```python
from build123d import *

# Parameters (mm, degrees)
BOSS_EXTRUDE1_DEPTH = 24
SKETCH2_R           = 10.5
CUT_EXTRUDE1_DEPTH  = 2.5
SKETCH4_R           = 2.25
SKETCH4_R_2         = 1.25
CUT_EXTRUDE2_DEPTH  = 10
SKETCH11_R          = 3
BOSS_EXTRUDE2_DEPTH = 4
CUT_EXTRUDE5_DEPTH  = 65
SKETCH13_W          = 24
SKETCH13_H          = 8.6
SKETCH13_R          = 2.2
BOSS_EXTRUDE3_DEPTH = 5
SKETCH14_W          = 5
SKETCH14_H          = 15
BOSS_EXTRUDE4_DEPTH = 7.5
SKETCH15_W          = 3
SKETCH15_H          = 15
BOSS_EXTRUDE5_DEPTH = 20
SKETCH16_R          = 5.05
CUT_EXTRUDE6_DEPTH  = 79.900823823
CHAMFER1_SIZE       = 3
CHAMFER2_SIZE       = 1
FILLET2_R           = 6
FILLET7_R           = 3
FILLET8_R           = 0.5


with BuildPart() as part:
    # Sketch1 → Boss-Extrude1 (new body)
    with BuildSketch(Plane(origin=(0, 0, 0), x_dir=(0, 0, -1), z_dir=(1, 0, 0))):
        Polygon((0, 59.7), (0, 0), (-43, 0), (-43, 5), (-8.535533906, 5), (-5, 8.535533906), (-5, 51.164466094), (-8.535533906, 54.7), (-43, 54.7), (-43, 59.7), align=None)
    extrude(amount=BOSS_EXTRUDE1_DEPTH)

    # Sketch2 → Cut-Extrude1 (cut)
    with BuildSketch(Plane.XZ.offset(-54.7)):
        with Locations(Location((12, 31, 0), (0, 0, 270))):
            Circle(SKETCH2_R)
    extrude(amount=-CUT_EXTRUDE1_DEPTH, mode=Mode.SUBTRACT)

    # Sketch4 → Cut-Extrude2 (cut)
    with BuildSketch(Plane.XZ.offset(-57.2)):
        with Locations(Location((12, 31, 0), (0, 0, 270))):
            Circle(SKETCH4_R)
        with Locations(Location((12, 38.25, 0), (0, 0, 270))):
            Circle(SKETCH4_R_2)
        with Locations(Location((8.5, 38.25, 0), (0, 0, 270))):
            Circle(SKETCH4_R_2)
        with Locations(Location((15.5, 38.25, 0), (0, 0, 270))):
            Circle(SKETCH4_R_2)
        with Locations(Location((19.25, 34.5, 0), (0, 0, 270))):
            Circle(SKETCH4_R_2)
        with Locations(Location((19.25, 31, 0), (0, 0, 270))):
            Circle(SKETCH4_R_2)
        with Locations(Location((19.25, 27.5, 0), (0, 0, 270))):
            Circle(SKETCH4_R_2)
        with Locations(Location((15.5, 23.75, 0), (0, 0, 270))):
            Circle(SKETCH4_R_2)
        with Locations(Location((12, 23.75, 0), (0, 0, 270))):
            Circle(SKETCH4_R_2)
        with Locations(Location((8.5, 23.75, 0), (0, 0, 270))):
            Circle(SKETCH4_R_2)
        with Locations(Location((4.75, 27.5, 0), (0, 0, 270))):
            Circle(SKETCH4_R_2)
        with Locations(Location((4.75, 31, 0), (0, 0, 270))):
            Circle(SKETCH4_R_2)
        with Locations(Location((4.75, 34.5, 0), (0, 0, 270))):
            Circle(SKETCH4_R_2)
    extrude(amount=-CUT_EXTRUDE2_DEPTH, mode=Mode.SUBTRACT)

    # Sketch11 → Boss-Extrude2 (add)
    with BuildSketch(Plane(origin=(0, 5, 0), x_dir=(1, 0, 0), z_dir=(0, 1, 0))):
        with Locations(Location((12, -31, 0), (0, 0, 90))):
            Circle(SKETCH11_R)
    extrude(amount=BOSS_EXTRUDE2_DEPTH)

    # Sketch12 → Cut-Extrude5 (cut, symmetric)
    with BuildSketch(Plane.XZ.offset(-54.7)):
        with BuildLine():
            Line((6, 12.017766953), (18, 12.017766953))
            ThreePointArc((18, 12.017766953), (20.5, 14.517766953), (18, 17.017766953))
            Line((18, 17.017766953), (6, 17.017766953))
            ThreePointArc((6, 17.017766953), (3.5, 14.517766953), (6, 12.017766953))
        make_face()
    extrude(amount=CUT_EXTRUDE5_DEPTH, both=True, mode=Mode.SUBTRACT)

    # Sketch13 → Boss-Extrude3 (add)
    # profile 1 of 2: a face of its own
    with BuildSketch(Plane.ZY):
        with Locations((-12, 4.3)):
            Rectangle(SKETCH13_W, SKETCH13_H)
        with Locations((-16.95, 4.3)):
            Circle(SKETCH13_R, mode=Mode.SUBTRACT)
        with Locations((-7.05, 4.3)):
            Circle(SKETCH13_R, mode=Mode.SUBTRACT)
    # profile 2 of 2: a face of its own
    with BuildSketch(Plane.ZY):
        with Locations((-12, 53.4)):
            Rectangle(SKETCH13_W, SKETCH13_H)
        with Locations(Location((-16.95, 53.4, 0), (0, 0, 180))):
            Circle(SKETCH13_R, mode=Mode.SUBTRACT)
        with Locations(Location((-7.05, 53.4, 0), (0, 0, 180))):
            Circle(SKETCH13_R, mode=Mode.SUBTRACT)
    extrude(amount=-BOSS_EXTRUDE3_DEPTH)

    # Sketch14 → Boss-Extrude4 (add)
    with BuildSketch(Plane(origin=(24, 0, 0), x_dir=(0, 0, -1), z_dir=(1, 0, 0))):
        with Locations((-2.5, 17.6)):
            Rectangle(SKETCH14_W, SKETCH14_H)
    extrude(amount=BOSS_EXTRUDE4_DEPTH)

    # Sketch15 → Boss-Extrude5 (add)
    with BuildSketch(Plane(origin=(0, 0, 0), x_dir=(-1, 0, 0), z_dir=(0, 0, -1))):
        with Locations((-30, 17.6)):
            Rectangle(SKETCH15_W, SKETCH15_H)
    extrude(amount=BOSS_EXTRUDE5_DEPTH)

    # Sketch16 → Cut-Extrude6 (cut, through all)
    with BuildSketch(Plane.ZY.offset(-28.5)):
        with Locations((-12, 17.6)):
            Circle(SKETCH16_R)
    extrude(amount=-CUT_EXTRUDE6_DEPTH, mode=Mode.SUBTRACT)

    # Chamfer1
    chamfer1_edges = [part.edges().sort_by_distance(p)[0] for p in [
        (24, 25.1, 2.5),
    ]]
    chamfer(chamfer1_edges, length=CHAMFER1_SIZE)

    # Chamfer2
    chamfer2_edges = [part.edges().sort_by_distance(p)[0] for p in [
        (24, 10.1, 2.5),
    ]]
    chamfer(chamfer2_edges, length=CHAMFER2_SIZE)

    # Fillet2
    fillet2_edges = [part.edges().sort_by_distance(p)[0] for p in [
        (0, 2.5, 43),
        (0, 57.2, 43),
        (24, 2.5, 43),
        (24, 57.2, 43),
    ]]
    fillet(fillet2_edges, radius=FILLET2_R)

    # Fillet7
    # the kernel refuses this fillet: 3 mm, written as the material it takes off along each edge
    with BuildSketch(Plane(origin=(-7.5, 59.7, 0), x_dir=(0, -1, 0), z_dir=(1, 0, 0))) as fillet7_piece_1_section:
        with BuildLine():
            CenterArc((FILLET7_R, -FILLET7_R), FILLET7_R, 90, 90)
            Line((0, -FILLET7_R), (0, 0))
            Line((0, 0), (FILLET7_R, 0))
        make_face()
    fillet7_piece_1 = extrude(amount=39, mode=Mode.PRIVATE)
    fillet7_piece_1 = split(fillet7_piece_1, bisect_by=Plane(origin=(2.5, 57.7, 0.688760919), z_dir=(0, 1, 0)), keep=Keep.TOP, mode=Mode.PRIVATE)
    add(fillet7_piece_1, mode=Mode.SUBTRACT)
    with BuildSketch(Plane(origin=(-7.5, 59.7, 0), x_dir=(0, -1, 0), z_dir=(1, 0, 0))) as fillet7_piece_2_section:
        with BuildLine():
            CenterArc((FILLET7_R, -FILLET7_R), FILLET7_R, 90, 90)
            Line((0, -FILLET7_R), (0, 0))
            Line((0, 0), (FILLET7_R, 0))
        make_face()
    fillet7_piece_2 = extrude(amount=39, mode=Mode.PRIVATE)
    fillet7_piece_2 = split(fillet7_piece_2, bisect_by=Plane(origin=(5, 57.451452112, 0.051209323), z_dir=(1, 0, 0)), keep=Keep.TOP, mode=Mode.PRIVATE)
    add(fillet7_piece_2, mode=Mode.SUBTRACT)
    with BuildSketch(Plane(origin=(-7.5, 0, -24), x_dir=(0, 0, 1), z_dir=(1, 0, 0)), Plane(origin=(-7.5, 8.6, -24), x_dir=(0, -1, 0), z_dir=(1, 0, 0)), Plane(origin=(-7.5, 49.1, -24), x_dir=(0, 0, 1), z_dir=(1, 0, 0))) as fillet7_piece_3:
        with BuildLine():
            CenterArc((FILLET7_R, -FILLET7_R), FILLET7_R, 90, 90)
            Line((0, -FILLET7_R), (0, 0))
            Line((0, 0), (FILLET7_R, 0))
        make_face()
    extrude(amount=20, mode=Mode.SUBTRACT)
    with BuildSketch(Plane(origin=(-7.5, 57.7, -24), x_dir=(0, 0, 1), z_dir=(1, 0, 0))) as fillet7_piece_4:
        with BuildLine():
            CenterArc((FILLET7_R, FILLET7_R), FILLET7_R, 180, 90)
            Line((0, FILLET7_R), (0, 0))
            Line((0, 0), (FILLET7_R, 0))
        make_face()
    extrude(amount=20, mode=Mode.SUBTRACT)
    with BuildSketch(Plane(origin=(31.5, 32.6, 5), x_dir=(-1, 0, 0), z_dir=(0, -1, 0))) as fillet7_piece_5:
        with BuildLine():
            CenterArc((FILLET7_R, FILLET7_R), FILLET7_R, 180, 90)
            Line((0, FILLET7_R), (0, 0))
            Line((0, 0), (FILLET7_R, 0))
        make_face()
    extrude(amount=30, mode=Mode.SUBTRACT)
    with BuildSketch(Plane(origin=(21, 10.1, -20), x_dir=(0, 0, 1), z_dir=(1, 0, 0)), Plane(origin=(39, 25.1, -20), x_dir=(0, 0, 1), z_dir=(-1, 0, 0))) as fillet7_piece_6:
        with BuildLine():
            CenterArc((FILLET7_R, -FILLET7_R), FILLET7_R, 90, 90)
            Line((0, -FILLET7_R), (0, 0))
            Line((0, 0), (FILLET7_R, 0))
        make_face()
    extrude(amount=18, mode=Mode.SUBTRACT)
    with BuildSketch(Plane(origin=(5, 0, 0), x_dir=(0, 0, 1), z_dir=(1, 0, 0))) as fillet7_piece_7:
        with BuildLine():
            CenterArc((FILLET7_R, -FILLET7_R), FILLET7_R, 90, 90)
            Line((0, -FILLET7_R), (0, 0))
            Line((0, 0), (FILLET7_R, 0))
        make_face()
    extrude(amount=26.5, mode=Mode.SUBTRACT)

    # Fillet8
    fillet8_edges = [part.edges().sort_by_distance(p)[0] for p in [
        (12, 9, 34),
    ]]
    fillet(fillet8_edges, radius=FILLET8_R)


solid = part.part
```
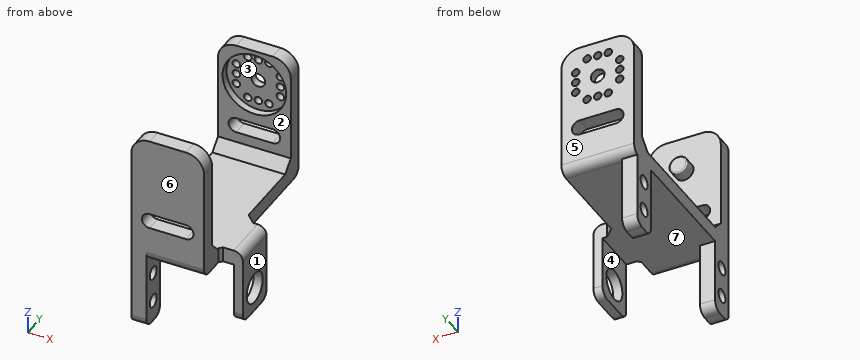
Design review of the part built by this model. Coordinates are the model's own, in mm. Face numbers are marked on the shaded views. A direction names the side the tool comes from. Round coordinates to 2 decimals unless told otherwise and drop trailing zeros. Order: outer loops, then holes, each group sorted by start corner. A loop starts at its lowest first (then second) coordinate and runs counter-clockwise, first axis right, second up. Notation, with made-up numbers: M 27.25,75.25 L 73.25,75.25 A20 cw 73.25,109.25 Z; hole C 31,7 d11. An arc over 180 degrees is marked long. Put each result on its own line as item: value.
Q1. Consider section B-B (z = -12). State the section outline as (x, y) points.
Reported:
outline: M 0,0 L 5,0 L 5,8.6 L 0,8.6 Z; M 0,49.1 L 5,49.1 L 5,57.7 L 0,57.7 Z; M 28.5,10.1 L 31.5,10.1 L 31.5,12.55 L 28.5,12.55 Z; M 28.5,22.65 L 31.5,22.65 L 31.5,25.1 L 28.5,25.1 Z
Q2. Consider section A-A (z = 31). State how many separate pieces and enclosed holes the cut face has, and give its area (3 significant figures).
Reported:
separate pieces: 5
enclosed holes: 0
area: 188 mm²
Q3. Draft analysis for pull direction Y (two halves, no side actions). For the marked faces 4, 5, 6 and 7, state which applies: released by +Y, released by -Y, zero draft, split by the parting line, or undercut.
Reported:
face 4: zero draft
face 5: released by +Y
face 6: released by -Y
face 7: undercut
Q4. To check wall thickness, follow line 1 (Z direction, x = 3.05, y = 53.4); line 2 (X direction, y = 58, z = 38); line 3 (Y direction, x = 17, z = 40.5). State the ranges of each line that lie inside material, in increasing order.
Reported:
line 1: -24 to -19.15, -14.75 to -9.25, -4.85 to 7.24
line 2: 0.08 to 7.28, 9.72 to 10.78, 13.22 to 14.28, 16.72 to 23.92
line 3: 0 to 5, 54.7 to 59.7
Q5. Machinability: for the marked faces 1, 2 and 3, which of the approach directions +Z, -Z, +X, -X, +Y, -Y give a long, thin tool a straight path to every point of the face, cutting with its end or side? Answer none if there is none.
Reported:
face 1: +Z, -Z, +X, +Y, -Y
face 2: +Z, +X, -X
face 3: none
Q6. Insertion check: pin 1 Ø7 at (y, z) = (53.4, -7.05) entering from -X; pin 2 Ø4 at (x, y) = (6, 22.5) entering from +Z; pin 3 Ø1.5 at (x, z) = (12, 31) entering from +Y; pin 4 Ø1.5 at (x, y) = (8.5, 50.5) entering from -Z. Each pin has a flat end and moves straight along its axis. Give the tip position at first contact, or say it passes through.
Reported:
pin 1: x = 0
pin 2: z = 5
pin 3: y = 9
pin 4: z = 0
Q7. Consider section C-C (y = 21). State the section outline as (x, z) points, and give its area (3 significant figures).
Reported:
outline: M 0,0 L 28.5,0 L 28.5,-8.27 L 31.5,-8.27 L 31.5,2 A3 ccw 28.5,5 L 0,5 Z; M 28.5,-20 L 31.5,-20 L 31.5,-15.73 L 28.5,-15.73 Z
area: 193 mm²
